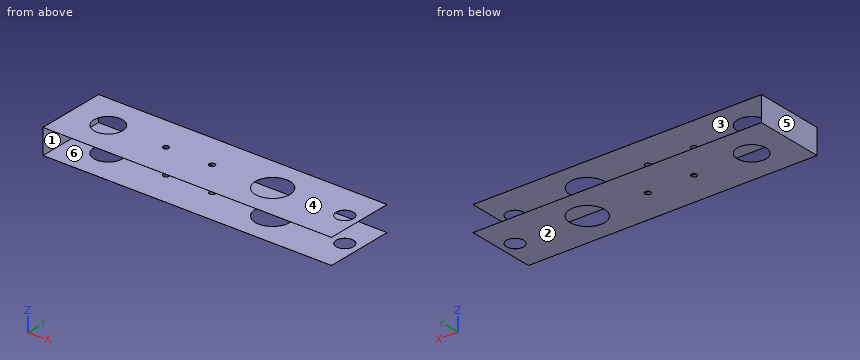
```python
from build123d import *

# Parameters (mm, degrees)
EXTRUDE_1_DEPTH     = 120
SKETCH_2_R          = 25
SKETCH_2_R_2        = 5
SKETCH_2_R_3        = 30
SKETCH_2_R_4        = 15
CUT_EXTRUDE_1_DEPTH = 120


with BuildPart() as part:
    # 草图1 → 凸台-拉伸1 (new body)
    with BuildSketch(Plane(origin=(0, 0, 0), x_dir=(1, 0, 0), z_dir=(0, 1, 0))):
        Polygon((815.722184809, 138.335459402), (315.622184809, 138.335459402), (315.622184809, 95.135459402), (815.722184809, 95.135459402), (815.722184809, 95.235459402), (315.722184809, 95.235459402), (315.722184809, 138.235459402), (815.722184809, 138.235459402), align=None)
    extrude(amount=EXTRUDE_1_DEPTH)

    # 草图2 → 切除-拉伸1 (cut)
    with BuildSketch(Plane(origin=(0, 0, -138.335459402), x_dir=(-1, 0, 0), z_dir=(0, 0, -1))):
        with Locations((-380.622184809, 60)):
            Circle(SKETCH_2_R)
        with Locations((-480.622184809, 60)):
            Circle(SKETCH_2_R_2)
        with Locations((-560.622184809, 60)):
            Circle(SKETCH_2_R_2)
        with Locations((-665.622184809, 60)):
            Circle(SKETCH_2_R_3)
        with Locations((-790.722184809, 60)):
            Circle(SKETCH_2_R_4)
    extrude(amount=-CUT_EXTRUDE_1_DEPTH, mode=Mode.SUBTRACT)


solid = part.part
```
Input: part model. Units: mm. Frame: model coordinates. Face numbers are marked on the shaded views. A direction names the side the tool comes from. Round coordinates to 2 decimals unless told otherwise and drop trailing zeros. Loops run counter-clockwise (first coordinate to the right, second up) from the corner with the lowest first, then second, coordinate; pieces in that order, holes last. Notation, with made-up numbers: (54, -12) -> (77, -12) arc R29 ccw to (77, 14) -> close; hole circle Ø5 at (32.5, 59). An arc over 180 degrees is marked (long way). Use one line per item in the form item = value. Start each with the question number.
Item 1: Mould query, pull axis Z, two halves, no side actions, for the marked faces 1, 2, 3 and 4. Classes: pulls with the +Z half, pulls with the -Z half, needs draft (parallel to the pull), parting line crosses it, or undercut.
Item 2: Section query C-C on z = -117.5. Return the cut outline in (x, y).
Item 3: Section query A-A on x = 504. Return the cut outline in (y, z), then the cut area to 3 significant figures.
Item 4: Contact query for flat-ended pins moving along their axis: pin 1 Ø4 at (y, z) = (14.5, -108.5) entering from +X; pin 2 Ø8 at (x, y) = (560.62, 60) entering from +Z (3 decimals). Output: stop coordinate, or through.
Item 5: Set-up query: the marked faces 5 and 6. Return all of +Z, -Z, +X, -X, +Y, -Y with unobstructed straight access to the full face (end or side cutting, diameter ignored); none if empty.
Item 6: Section query B-B on y = 14.5. Return the cut outline in (x, z), then the cut area to 3 significant figures.
Item 7: Section query D-D on y = 60. Count the separate pieces of the cut face and the enclosed holes in it, then the cut area to 3 significant figures.
Ans:
q1.face_1 = undercut
q1.face_2 = pulls with the -Z half
q1.face_3 = undercut
q1.face_4 = pulls with the +Z half
q2.outline = (315.62, 0) -> (315.72, 0) -> (315.72, 120) -> (315.62, 120) -> close
q3.outline = (0, -138.34) -> (120, -138.34) -> (120, -138.24) -> (0, -138.24) -> close; (0, -95.24) -> (120, -95.24) -> (120, -95.14) -> (0, -95.14) -> close
q3.area = 24.0 mm^2
q4.pin_1 = 315.72
q4.pin_2 = through
q5.face_5 = +Z, -Z, -X, +Y, -Y
q5.face_6 = +X, +Y, -Y
q6.outline = (315.62, -138.34) -> (815.72, -138.34) -> (815.72, -138.24) -> (315.72, -138.24) -> (315.72, -95.24) -> (815.72, -95.24) -> (815.72, -95.14) -> (315.62, -95.14) -> close
q6.area = 104 mm^2
q7.separate_pieces = 11
q7.enclosed_holes = 0
q7.area = 72.3 mm^2
